```python
from build123d import *

# Parameters (mm, degrees)
SKETCH2_W    = 0.75
SKETCH2_H    = 1
FILLET1_R    = 0.25
SCALE1_SCALE = 10


with BuildPart() as part:
    # Sweep1: sweep along a path in Sketch1
    with BuildLine(Plane(origin=(0, 0, 0), x_dir=(1, 0, 0), z_dir=(0, 1, 0))) as sweep1_path:
        Line((-3.95, 0), (-3.95, 13))
        ThreePointArc((-3.95, 13), (-3.364213562, 14.414213562), (-1.95, 15))
        Line((-1.95, 15), (1.95, 15))
        ThreePointArc((1.95, 15), (3.364213562, 14.414213562), (3.95, 13))
        Line((3.95, 13), (3.95, 0))
    # Sketch2 → Sweep1 (sweep)
    with BuildSketch(Plane.XY):
        with Locations((-4.325, 0.5)):
            Rectangle(SKETCH2_W, SKETCH2_H)
    sweep(path=sweep1_path.line)

    # Fillet1
    fillet1_edges = [part.edges().sort_by_distance(p)[0] for p in [
        (3.95, 1, -6.5),
        (4.7, 1, -6.5),
        (4.7, 0, -6.5),
        (-3.95, 0, -6.5),
        (-3.95, 1, -6.5),
        (-4.7, 1, -6.5),
        (-4.7, 0, -6.5),
        (-3.364213562, 0, -14.414213562),
        (-3.364213562, 1, -14.414213562),
        (-3.894543648, 1, -14.944543648),
        (-3.894543648, 0, -14.944543648),
        (0, 0, -15),
        (0, 1, -15),
        (0, 1, -15.75),
        (0, 0, -15.75),
        (3.364213562, 0, -14.414213562),
        (3.364213562, 1, -14.414213562),
        (3.894543648, 1, -14.944543648),
        (3.894543648, 0, -14.944543648),
        (3.95, 0, -6.5),
    ]]
    fillet(fillet1_edges, radius=FILLET1_R)


with BuildPart() as part_1:
    # Scale1: scaled about (0, 0.5, -9.028741483)
    add(part.part.scale(SCALE1_SCALE).moved(Location((0, -4.5, 81.258673347))))


solid = part_1.part
```
Here's how the part is built. I have some questions about the finished solid (model axes, mm). A direction names the side the tool comes from. Coordinates: 2 decimals unless noted, no trailing zeros. Order: outer loops, then holes, each group sorted by start corner. A loop starts at its lowest first (then second) coordinate and runs counter-clockwise, first axis right, second up. Notation, with made-up numbers: (-18.5, 88.25) - (-9.5, 88.25) arc R28 cw to (-9.5, 115.25) - close; hole circle Ø5 at (63.25, 12.5). An arc over 180 degrees is marked (long way). One line per question, with ' | ' between items. Start each with the question number.
1. If we section it at C-C (x = 0.5): Write out the boundary of the cut face in (y, z), and give its area (3 significant figures).
2. If we section it at A-A (z = 23.5): Write out the boundary of the cut face in (x, y), and give its area (3 significant figures).
3. I'm going to push a flat-ended pin straight in: pin 1 Ø2.5 at (x, y) = (-3, 1) entering from +Z. Where does the tip first touch, or does it pass through?
4. If we section it at B-B (y = 0.75): Write out the boundary of the cut face in (x, z), and give its area (3 significant figures).
5. Which directions (+Z, -Z, +X, -X, +Y, -Y) give clear straight access to the entire face, cutting with the end or side of a thin tool? Please do faces 4 (the flat face through (-43, -4.5, -2)), 5 (the cylindrical face through (33.486, 0.535, -63.038)).
6. If we mould it in two halves opening along X, with no side actions, what happens to faces 1 (the flat face through (-43, 1, 81.259)), 2 (the flat face through (0, 0, -68.741)), 3 (the cylindrical face through (38.73, 0.46, -68.4))? For each: released by +X, released by -X, zero draft, split by the parting line, or undercut.
7. Please list where these lines run through material, in increasing order: line 1 along X through (y, z) = (-2.25, 69); line 2 along Z through (x, y) = (10, -0.25); line 3 along X through (y, z) = (-1, -58). Write a range as [from, to].
Model answer:
1) outline: (-4.5, -73.74) arc R2.5 ccw to (-2, -76.24) - (3, -76.24) arc R2.5 ccw to (5.5, -73.74) - (5.5, -71.24) arc R2.5 ccw to (3, -68.74) - (-2, -68.74) arc R2.5 ccw to (-4.5, -71.24) - close | area: 69.6 mm²
2) outline: (-47, -2) arc R2.5 ccw to (-44.5, -4.5) - (-42, -4.5) arc R2.5 ccw to (-39.5, -2) - (-39.5, 3) arc R2.5 ccw to (-42, 5.5) - (-44.5, 5.5) arc R2.5 ccw to (-47, 3) - close; (39.5, -2) arc R2.5 ccw to (42, -4.5) - (44.5, -4.5) arc R2.5 ccw to (47, -2) - (47, 3) arc R2.5 ccw to (44.5, 5.5) - (42, 5.5) arc R2.5 ccw to (39.5, 3) - close | area: 139 mm²
3) pin 1: stops at z = -68.74
4) outline: (-47, -48.74) arc R27.5 ccw to (-19.5, -76.24) - (19.5, -76.24) arc R27.5 ccw to (47, -48.74) - (47, 81.26) - (39.5, 81.26) - (39.5, -48.74) arc R20 cw to (19.5, -68.74) - (-19.5, -68.74) arc R20 cw to (-39.5, -48.74) - (-39.5, 81.26) - (-47, 81.26) - close | area: 2,800 mm²
5) face 4: +Z, -Z, +X, -X, -Y | face 5: +Z, +Y, -Y
6) face 1: zero draft | face 2: undercut | face 3: released by +X
7) line 1: x = [-46.99, -39.51], [39.51, 46.99] | line 2: z = [-76.24, -68.74] | line 3: x = [-45.39, -37.23], [37.23, 45.39]
